The listing builds one solid part. Answer for the finished solid, in the listing's coordinates (mm). A direction names the side the tool comes from. Give positions to 0.01 mm unless a question says otherwise; leave off trailing zeros. Loops run counter-clockwise (first coordinate to the right, second up) from the corner with the lowest first, then second, coordinate; pieces in that order, holes last. Notation, with made-up numbers: (19.5, 87.5) - (66.5, 87.5) arc R35 ccw to (66.5, 123.5) - close; hole circle Ø5 at (52.5, -4.5). An arc over 180 degrees is marked (long way). One line per item, written item: value. Start each with the question number.
from build123d import *

# Parameters (mm, degrees)
SKETCH1_W                                           = 52
SKETCH1_H                                           = 52
BOSS_EXTRUDE1_DEPTH                                 = 5
CBORE_FOR_2_BINDING_HEAD_MACHINE_SCREW1_D           = 2.4384
CBORE_FOR_2_BINDING_HEAD_MACHINE_SCREW1_CBORE_D     = 5.55752
CBORE_FOR_2_BINDING_HEAD_MACHINE_SCREW1_CBORE_DEPTH = 1.27


with BuildPart() as part:
    # Sketch1 → Boss-Extrude1 (new body)
    with BuildSketch(Plane(origin=(0, 0, 0), x_dir=(0, 0, -1), z_dir=(1, 0, 0))):
        with Locations((26, 26)):
            Rectangle(SKETCH1_W, SKETCH1_H)
    extrude(amount=BOSS_EXTRUDE1_DEPTH)

    # CBORE for #2 Binding Head Machine Screw1 (through all)
    with Locations(Plane(origin=(5, 0, 0), x_dir=(0, 0, -1), z_dir=(1, 0, 0))):
        with Locations((13, 49.5), (39, 49.5), (49.5, 39), (49.5, 13), (39, 2.5), (13, 2.5), (2.5, 13), (2.5, 39)):
            CounterBoreHole(CBORE_FOR_2_BINDING_HEAD_MACHINE_SCREW1_D / 2, CBORE_FOR_2_BINDING_HEAD_MACHINE_SCREW1_CBORE_D / 2, CBORE_FOR_2_BINDING_HEAD_MACHINE_SCREW1_CBORE_DEPTH)


solid = part.part
1. A cutting plane is placed at A-A (y = 13). Determine the outline of the cut face in (x, z).
2. A flat-ended cylindrical pin translates along its axis: pin 1 (2.5 mm diameter, centred on y = 39, z = -3, fed in from +X). Find the tip coordinate at first contact, or state that the pin passes through.
3. Find the intervals of material crossed by L1, parallel to Y at x = 4.15, z = -49.5; L2, parallel to Y at x = 3.6, z = -39; L3, parallel to X at y = 15.5, z = -3, in increasing order. Write a range as [from, to].
4. A cutting plane is placed at C-C (y = 2.5). Determine the outline of the cut face in (x, z), plus the area to 3 significant figures.
5. Determine the mould class of faces 1 (the flat face through (5, 26, -26)), 2 (the flat face through (2, 0, -26)), 3 (the cylindrical face through (1.8, 1.8, -14)), 4 (the cylindrical face through (1.84, 49.87, -37.84)) for opening direction Y: released by +Y, released by -Y, zero draft, split by the parting line, or undercut.
6. For faces 5 (the cylindrical face through (1.84, 37.81, -2.76)), 6 (the cylindrical face through (4.374, 12.895, -5.277)), determine the directions among +Z, -Z, +X, -X, +Y, -Y from which every point of the face is accessible in a straight line to the end or side of a thin tool.
7. A cutting plane is placed at B-B (z = -39). Determine the outline of the cut face in (x, y).
8. A cutting plane is placed at D-D (z = -2.5). Determine the outline of the cut face in (x, y).
Results below:
1. outline: (0, -52) - (3.73, -52) - (3.73, -50.72) - (0, -50.72) - close; (0, -48.28) - (3.73, -48.28) - (3.73, -46.72) - (5, -46.72) - (5, -5.28) - (3.73, -5.28) - (3.73, -3.72) - (0, -3.72) - close; (0, -1.28) - (3.73, -1.28) - (3.73, 0) - (0, 0) - close
2. pin 1: stops at x = 3.73
3. L1: y = [0, 10.22], [15.78, 36.22], [41.78, 52]
3. L2: y = [0, 1.28], [3.72, 48.28], [50.72, 52]
3. L3: x = [0, 3.73]
4. outline: (0, -52) - (5, -52) - (5, -41.78) - (3.73, -41.78) - (3.73, -40.22) - (0, -40.22) - close; (0, -37.78) - (3.73, -37.78) - (3.73, -36.22) - (5, -36.22) - (5, -15.78) - (3.73, -15.78) - (3.73, -14.22) - (0, -14.22) - close; (0, -11.78) - (3.73, -11.78) - (3.73, -10.22) - (5, -10.22) - (5, 0) - (0, 0) - close
4. area: 228 mm^2
5. face 1: zero draft
5. face 2: released by -Y
5. face 3: undercut
5. face 4: undercut
6. face 5: +X, -X
6. face 6: +X
7. outline: (0, 0) - (3.73, 0) - (3.73, 1.28) - (0, 1.28) - close; (0, 3.72) - (3.73, 3.72) - (3.73, 5.28) - (5, 5.28) - (5, 46.72) - (3.73, 46.72) - (3.73, 48.28) - (0, 48.28) - close; (0, 50.72) - (3.73, 50.72) - (3.73, 52) - (0, 52) - close
8. outline: (0, 0) - (5, 0) - (5, 10.22) - (3.73, 10.22) - (3.73, 11.78) - (0, 11.78) - close; (0, 14.22) - (3.73, 14.22) - (3.73, 15.78) - (5, 15.78) - (5, 36.22) - (3.73, 36.22) - (3.73, 37.78) - (0, 37.78) - close; (0, 40.22) - (3.73, 40.22) - (3.73, 41.78) - (5, 41.78) - (5, 52) - (0, 52) - close
